```python
from build123d import *

# Parameters (mm, degrees)
F1_DEPTH = 100
F2_R     = 4
F2_R_2   = 3
F3_DEPTH = 100


with BuildPart() as f1:
    # F0 (on Front) → F1 (new body)
    with BuildSketch(Plane.XZ):
        Polygon((5.189254, 40), (5.189254, 0), (5.189254, -40), (30.189254, -40), (30.189254, -8), (55.189254, -8), (55.189254, 8), (30.189254, 8), (30.189254, 40), align=None)
    extrude(amount=F1_DEPTH)

    # F2 (on face) → F3 (cut)
    with BuildSketch(Plane(origin=(5.189254, 0, 0), x_dir=(0, -1, 0), z_dir=(-1, 0, 0))):
        with Locations((25, 25)):
            Circle(F2_R)
        with Locations((75, 25)):
            Circle(F2_R)
        with Locations((25, -25)):
            Circle(F2_R)
        with Locations((75, -25)):
            Circle(F2_R)
        with Locations((15, 35)):
            Circle(F2_R_2)
        with Locations((85, 35)):
            Circle(F2_R_2)
        with Locations((15, -35)):
            Circle(F2_R_2)
        with Locations((85, -35)):
            Circle(F2_R_2)
    extrude(amount=-F3_DEPTH, mode=Mode.SUBTRACT)


solid = f1.part
```
Could you check a few things on this model? Use its own coordinates, in mm. A direction names the side the tool comes from. Coordinates: 2 decimals unless noted, no trailing zeros. Loops run counter-clockwise (first coordinate to the right, second up) from the corner with the lowest first, then second, coordinate; pieces in that order, holes last. Notation, with made-up numbers: M 68,61.5 L 106,61.5 A14 ccw 106,78.5 Z; hole C -12.75,32.25 d7. An arc over 180 degrees is marked long. Put each result on its own line as item: value. Start each with the question number.
(1) Suppose I cut it at B-B on y = -15. Please give me the cut outline in (x, z).
(2) Thinking about a two-plate mould opening in Y: for faces 4 (the face through (19, 0, 1)), 5 (the face through (5.189, -49, 1)), 6 (the face through (18, -82, -35)), which applies, pulls with the +Y half, pulls with the -Y half, needs draft (parallel to the pull), parting line crosses it, or undercut?
(3) Suppose I cut it at D-D on y = -25. Please give me the cut outline in (x, z), then the cut area to 3 significant figures.
(4) I need wall thicknesses on line 1 (Z direction, x = 25.25, y = -75); line 2 (Z direction, x = 22.75, y = -85); line 3 (Y direction, x = 9, z = -27.5). Which ranges of each line are inside material? Lowest first, please. Write a range as from..to.
(5) Suppose I cut it at C-C on x = 29. Count the separate pieces of the cut face and the enclosed holes in it, then the cut area to 3 significant figures.
(6) For faces 1 (the face through (55.189, -49, 0)), 2 (the face through (30.189, -49, -24)), 3 (the face through (43, -49, 8)), which set-ups out of +Z, -Z, +X, -X, +Y, -Y let a thin tool reach every point of the face, with its end or its side?
(7) Will these pins go through, and if not, where does the flat tip stop? P1, Ø3.5, axis at y = -85, z = -35, coming from the -X side; P2, Ø12.5, axis at x = 38.5, y = -68, coming from the +Z side; P3, Ø9.5, axis at y = -42.5, z = 21.5, coming from the +X side; P4, Ø12.5, axis at x = 44, y = -44.5, coming from the -Z side.
(8) Suppose I cut it at A-A on z = -25. Please give me the cut outline in (x, y).
Solutions:
1. outline: M 5.19,-40 L 30.19,-40 L 30.19,-38 L 5.19,-38 Z; M 5.19,-32 L 30.19,-32 L 30.19,-8 L 55.19,-8 L 55.19,8 L 30.19,8 L 30.19,32 L 5.19,32 Z; M 5.19,38 L 30.19,38 L 30.19,40 L 5.19,40 Z
2. face 4: pulls with the +Y half
2. face 5: needs draft
2. face 6: undercut
3. outline: M 5.19,-40 L 30.19,-40 L 30.19,-29 L 5.19,-29 Z; M 5.19,-21 L 30.19,-21 L 30.19,-8 L 55.19,-8 L 55.19,8 L 30.19,8 L 30.19,21 L 5.19,21 Z; M 5.19,29 L 30.19,29 L 30.19,40 L 5.19,40 Z
3. area: 2,000 mm2
4. line 1: z = -40..-29, -21..21, 29..40
4. line 2: z = -40..-38, -32..32, 38..40
4. line 3: y = -100..-78.12, -71.88..-28.12, -21.88..0
5. separate pieces: 1
5. enclosed holes: 8
5. area: 7,690 mm2
6. face 1: +Z, -Z, +X, +Y, -Y
6. face 2: -Z, +X, +Y, -Y
6. face 3: +Z, +X, +Y, -Y
7. P1: passes through
7. P2: stops at z = 8
7. P3: stops at x = 30.19
7. P4: stops at z = -8
8. outline: M 5.19,-100 L 30.19,-100 L 30.19,-79 L 5.19,-79 Z; M 5.19,-71 L 30.19,-71 L 30.19,-29 L 5.19,-29 Z; M 5.19,-21 L 30.19,-21 L 30.19,0 L 5.19,0 Z
